from build123d import *

# Parameters (mm, degrees)
SKETCH_1_W          = 75
SKETCH_1_H          = 57
SKETCH_1_R          = 2.25
SKETCH_1_R_2        = 0.9
SKETCH_1_R_3        = 0.55
SKETCH_1_R_4        = 0.5
SKETCH_1_R_5        = 1.75
EXTRUDE_1_DEPTH     = 2
SKETCH_2_R          = 0.4
CUT_EXTRUDE_1_DEPTH = 2
SKETCH_3_R          = 0.5
CUT_EXTRUDE_2_DEPTH = 2


with BuildPart() as part:
    # Эскиз1 → Вытянуть1 (new body)
    with BuildSketch(Plane.XY):
        Rectangle(SKETCH_1_W, SKETCH_1_H)
        with Locations((-33, 24)):
            Circle(SKETCH_1_R, mode=Mode.SUBTRACT)
        with Locations(Location((33, 24, 0), (0, 0, 180))):
            Circle(SKETCH_1_R, mode=Mode.SUBTRACT)
        with Locations((33, -24)):
            Circle(SKETCH_1_R, mode=Mode.SUBTRACT)
        with Locations(Location((-33, -24, 0), (0, 0, 180))):
            Circle(SKETCH_1_R, mode=Mode.SUBTRACT)
        with Locations((-16, -22)):
            Circle(SKETCH_1_R_2, mode=Mode.SUBTRACT)
        with Locations((-10.92, -22)):
            Circle(SKETCH_1_R_2, mode=Mode.SUBTRACT)
        with Locations((34.75, -3.12)):
            Circle(SKETCH_1_R_3, mode=Mode.SUBTRACT)
        with Locations((34.75, -0.58)):
            Circle(SKETCH_1_R_3, mode=Mode.SUBTRACT)
        with Locations((34.75, 1.96)):
            Circle(SKETCH_1_R_3, mode=Mode.SUBTRACT)
        with Locations((34.75, 4.5)):
            Circle(SKETCH_1_R_3, mode=Mode.SUBTRACT)
        with Locations((-5.84, -12.7)):
            Circle(SKETCH_1_R_4, mode=Mode.SUBTRACT)
        with Locations((-21.08, -12.7)):
            Circle(SKETCH_1_R_4, mode=Mode.SUBTRACT)
        with Locations((-33.25, 1.25)):
            Circle(SKETCH_1_R_5, mode=Mode.SUBTRACT)
        with Locations((1.25, 1.25)):
            Circle(SKETCH_1_R_5, mode=Mode.SUBTRACT)
    extrude(amount=EXTRUDE_1_DEPTH)

    # Эскиз2 → Вырез-Вытянуть1 (cut)
    with BuildSketch(Plane.XY.offset(2)):
        with Locations((-17.7, 20.5)):
            Circle(SKETCH_2_R)
        with Locations((16.75, -24.75)):
            Circle(SKETCH_2_R)
        with Locations((17, -6)):
            Circle(SKETCH_2_R)
        with Locations((17.25, 11.5)):
            Circle(SKETCH_2_R)
        with Locations((-10.96, 20.5)):
            Circle(SKETCH_2_R)
        with Locations((0.04, 20.5)):
            Circle(SKETCH_2_R)
        with Locations((-10.96, 25.5)):
            Circle(SKETCH_2_R)
        with Locations((0.04, 25.5)):
            Circle(SKETCH_2_R)
        with Locations((22.75, -20.65)):
            Circle(SKETCH_2_R)
        with Locations((26.25, -20.65)):
            Circle(SKETCH_2_R)
        with Locations((22.5, -3.72)):
            Circle(SKETCH_2_R)
        with Locations((26, -3.72)):
            Circle(SKETCH_2_R)
        with Locations((22.75, 13.75)):
            Circle(SKETCH_2_R)
        with Locations((26.25, 13.75)):
            Circle(SKETCH_2_R)
    extrude(amount=-CUT_EXTRUDE_1_DEPTH, mode=Mode.SUBTRACT)

    # Эскиз3 → Вырез-Вытянуть2 (cut)
    with BuildSketch(Plane.XY.offset(2)):
        with Locations((20.35, 19.5)):
            Circle(SKETCH_3_R)
        with Locations((25.35, 19.5)):
            Circle(SKETCH_3_R)
        with Locations((25.35, 22.5)):
            Circle(SKETCH_3_R)
        with Locations((20.35, 22.5)):
            Circle(SKETCH_3_R)
        with Locations((20.35, 2)):
            Circle(SKETCH_3_R)
        with Locations((25.35, 2)):
            Circle(SKETCH_3_R)
        with Locations((25.35, 5)):
            Circle(SKETCH_3_R)
        with Locations((20.35, 5)):
            Circle(SKETCH_3_R)
        with Locations((20.35, -14.5)):
            Circle(SKETCH_3_R)
        with Locations((25.35, -14.5)):
            Circle(SKETCH_3_R)
        with Locations((25.35, -11.5)):
            Circle(SKETCH_3_R)
        with Locations((20.35, -11.5)):
            Circle(SKETCH_3_R)
    extrude(amount=-CUT_EXTRUDE_2_DEPTH, mode=Mode.SUBTRACT)


solid = part.part
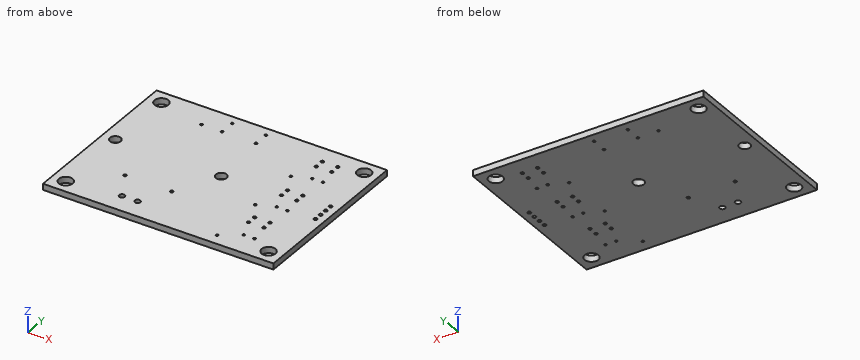
The listing builds one solid part. Answer for the finished solid, in the listing's coordinates (mm). Round coordinates to 2 decimals unless told otherwise and drop trailing zeros. Put each result on its own line as item: value.
Q1. Consider line 1 along X through (y, z) = (20.5, 0.9); line 2 along Y through (x, z) = (-10.96, 1.1); line 3 along Y through (x, z) = (17, 1.25). Determine where each line is inside the solid, lowest interval first.
Results list:
line 1: -37.5 to -18.1, -17.3 to -11.36, -10.56 to -0.36, 0.44 to 37.5
line 2: -28.5 to -22.9, -21.1 to 20.1, 20.9 to 25.1, 25.9 to 28.5
line 3: -28.5 to -25.06, -24.44 to -6.4, -5.6 to 11.19, 11.81 to 28.5
Q2. This flat-tipped pin is pushed along its axis until it touches: P1, Ø1.8, axis at x = 34.75, y = -3.12, coming from the +Z side. Where does it stop, or does it pass through?
Results list:
P1: z = 2
Q3. Section A-A, the plane z = 0.75 is taken. Count the separate pieces of the cut face and the enclosed holes in it, and give its area (3 significant figures).
Results list:
separate pieces: 1
enclosed holes: 40
area: 4,170 mm^2
